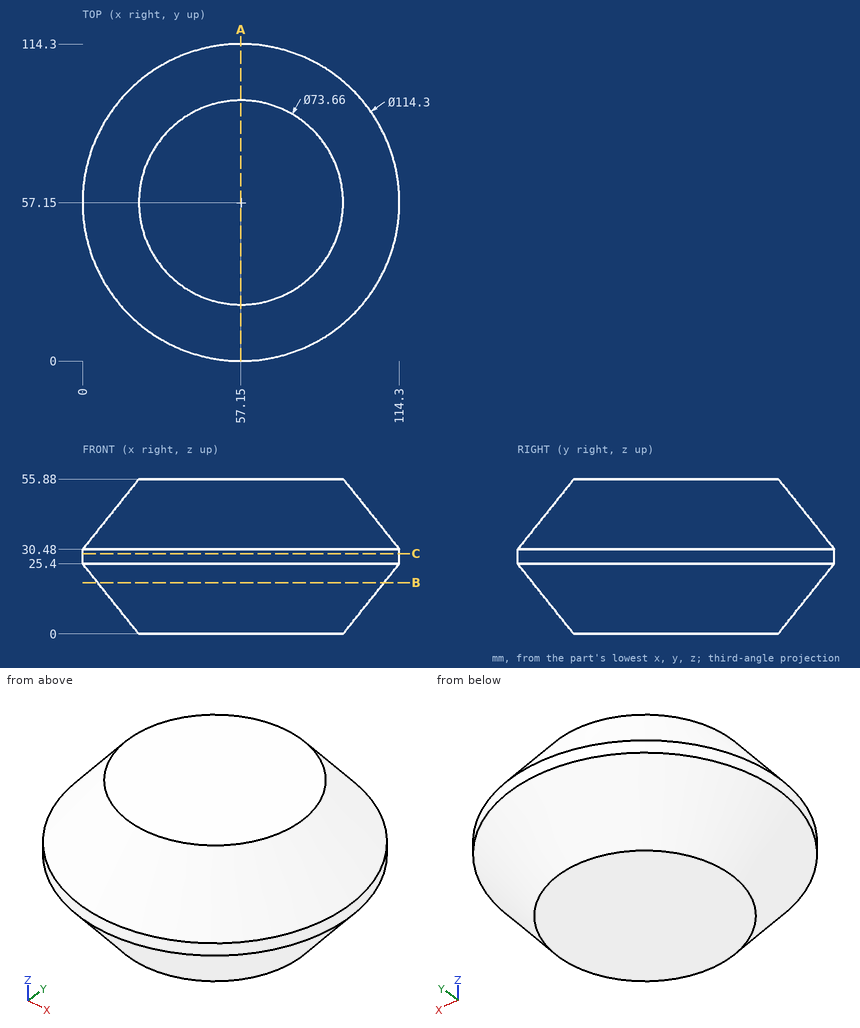
Input: dimensioned drawing with shaded views. Units: mm. Origin: part minimum x, y, z. Give positions to 0.01 mm unless a question says otherwise; leave off trailing zeros. Write each loop counter-clockwise with the first axis right and the second up, starting at its lowest first coordinate (ties: lowest second). Pieces come first, ordered by that corner, then holes. Notation, with made-up numbers: M 0,10.5 L 52,10.5 A24 ccw 52,26.5 Z; hole C -18.75,15 d9. An arc over 180 degrees is marked long. Return JSON: item names as keys, results as strings. Group by question number.
1) Pin query (flat end, axial travel): P1, Ø8, axis at y = 72.5, z = 33.5, coming from the -X side; P2, Ø1.5, axis at y = 56.5, z = 12, coming from the -X side; P3, Ø10, axis at x = 74, z = 38.5, coming from the -Y side. Return the tip coordinate at first contact, or that it passes through.
2) Cut plane A-A, the plane x = 57.15. Output: boundary loops of the cut face in (y, z).
3) Cut plane B-B, the plane z = 18.5. Output: boundary loops of the cut face in (x, y), plus the area to 3 significant figures.
4) Material intervals for line 1 along Z through (x, y) = (23, 74); line 2 along X through (y, z) = (82, 24); line 3 along X through (y, z) = (80.5, 22), sorted ascending. Write a range as [from, to].
5) Cut plane C-C, the plane z = 29. Output: boundary loops of the cut face in (x, y), plus the area to 3 significant figures.
Recorded:
{
 "1": {"P1": "stops at x = 1.44", "P2": "stops at x = 10.12", "P3": "stops at y = 4.8"},
 "2": {"outline": "M 0,25.4 L 20.32,0 L 93.98,0 L 114.3,25.4 L 114.3,30.48 L 93.98,55.88 L 20.32,55.88 L 0,30.48 Z"},
 "3": {"outline": "C 57.15,57.15 d103.26", "area": "8,370 mm²"},
 "4": {"line 1": "z = [1.56, 54.32]", "line 2": "x = [6.93, 107.37]", "line 3": "x = [7.98, 106.32]"},
 "5": {"outline": "C 57.15,57.15 d114.3", "area": "10,300 mm²"}
}
